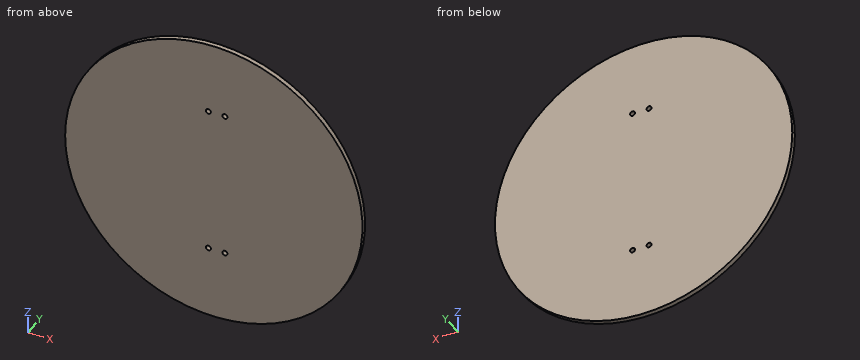
Autodesk Inventor part; units mm, degrees
ref_plane "YZ Plane" through (0, 0, 0) normal (1, 0, 0) x (0, 1, 0)
ref_plane "XZ Plane" through (0, 0, 0) normal (0, 1, 0) x (-1, 0, 0)
ref_plane "XY Plane" through (0, 0, 0) normal (0, 0, 1) x (1, 0, 0)
sketch "Sketch1" plane through (0, 0, 0) normal (0, 1, 0) x (-1, 0, 0)
  circle A0 centre (0, 0) radius 90
  line L0 (0, 0) -> (3.3, 0) construction
  line L1 (3.3, 0) -> (3.3, 45.5) construction
  circle A1 centre (3.3, 45.5) radius 1.5
  line L2 (3.3, 45.5) -> (-6.7, 45.5) construction
  circle A2 centre (-6.7, 45.5) radius 1.5
  line L3 (3.3, 0) -> (3.3, -45.5) construction
  circle A3 centre (3.3, -45.5) radius 1.5
  line L4 (3.3, -45.5) -> (-6.7, -45.5) construction
  circle A4 centre (-6.7, -45.5) radius 1.5
  dimension "d0" = 180
  dimension "d1" = 3.3
  dimension "d2" = 45.5
  dimension "d3" = 3
  dimension "d4" = 10
  dimension "d5" = 3
  dimension "d6" = 45.5
  dimension "d7" = 3
  dimension "d8" = 10
  dimension "d9" = 3
extrude "Extrusion1" add sketch "Sketch1" along normal blind 3
properties part number "hiago_tampassl2"
Model file for the job. Use its own axes, mm. Round coordinates to 2 decimals unless told otherwise and drop trailing zeros. Write each loop counter-clockwise with the first axis right and the second up, starting at its lowest first coordinate (ties: lowest second). Pieces come first, ordered by that corner, then holes. Notation, with made-up numbers: (7.5, 61) - (26.5, 61) arc R25 ccw to (26.5, 88) - close; hole circle Ø7 at (59, 7.5). An arc over 180 degrees is marked (long way). Use CSV: the item, a comma, the result in double quotes. Start each with the question number.
Item 1: Drill centre lines: L1, parallel to Z at x = 6.7, y = 1.5; L2, parallel to Z at x = -3.3, y = 1.9; L3, parallel to Z at x = 3, y = 1.2. Where is each one in solid material? Low to high. Write a range as [from, to].
Item 2: Band-saw the part on C-C (x = 61). Write the cut outline in (y, z), and give its area (3 significant figures).
Item 3: Band-saw the part on A-A (y = 1.85). Write the cut outline in (x, z), and give its area (3 significant figures).
Item 4: Band-saw the part on B-B (x = 43). Write the cut outline in (y, z), and give its area (3 significant figures).
Checked values:
1,L1,"z = [-89.75, -47], [-44, 44], [47, 89.75]"
1,L2,"z = [-89.94, -47], [-44, 44], [47, 89.94]"
1,L3,"z = [-89.95, 89.95]"
2,outline,"(0, -66.17) - (3, -66.17) - (3, 66.17) - (0, 66.17) - close"
2,area,"397 mm²"
3,outline,"circle Ø180 at (0, 0); hole circle Ø3 at (-3.3, -45.5); hole circle Ø3 at (-3.3, 45.5); hole circle Ø3 at (6.7, -45.5); hole circle Ø3 at (6.7, 45.5)"
3,area,"25,400 mm²"
4,outline,"(0, -79.06) - (3, -79.06) - (3, 79.06) - (0, 79.06) - close"
4,area,"474 mm²"
